from build123d import *

# Parameters (mm, degrees)
SKETCH_1_R          = 1.525
EXTRUDE_1_DEPTH     = 3.75
SKETCH_2_R          = 2.5
CUT_EXTRUDE_1_DEPTH = 10.5
CHAMFER_1_SIZE      = 3
SKETCH_3_R          = 2.5
CUT_EXTRUDE_2_DEPTH = 15.84082208
FILLET_1_R          = 0.5


with BuildPart() as part:
    # 草图1 → 凸台-拉伸1 (new, symmetric)
    with BuildSketch(Plane.XY):
        Polygon((-10, 8), (-10, -8), (6.931382282, -8), (10, -7), (10, 7), (6.931382282, 8), align=None)
        with Locations((0, 5)):
            Circle(SKETCH_1_R, mode=Mode.SUBTRACT)
        with Locations((0, -5)):
            Circle(SKETCH_1_R, mode=Mode.SUBTRACT)
    extrude(amount=EXTRUDE_1_DEPTH, both=True)

    # 草图2 → 切除-拉伸1 (cut)
    with BuildSketch(Plane.ZY.offset(10)):
        with Locations((4.25, 0)):
            Circle(SKETCH_2_R)
    extrude(amount=-CUT_EXTRUDE_1_DEPTH, mode=Mode.SUBTRACT)

    # 倒角1
    chamfer_1_edges = [part.edges().sort_by_distance(p)[0] for p in [
        (-10, -8, 0),
        (-10, 8, 0),
    ]]
    chamfer(chamfer_1_edges, length=CHAMFER_1_SIZE)

    # 草图3 → 切除-拉伸2 (cut, through all)
    with BuildSketch(Plane(origin=(0, 0, -3.75), x_dir=(-1, 0, 0), z_dir=(0, 0, -1))):
        with Locations((-10, 0)):
            Circle(SKETCH_3_R)
    extrude(amount=-CUT_EXTRUDE_2_DEPTH, mode=Mode.SUBTRACT)

    # 圆角1
    fillet_1_edges = [part.edges().sort_by_distance(p)[0] for p in [
        (6.931382282, 8, 0),
        (10, 7, 0),
        (10, -7, 0),
        (6.931382282, -8, 0),
        (-7, -8, 0),
        (-10, 5, 0),
        (-10, -5, 0),
        (-7, 8, 0),
        (10, -2.5, 0),
        (10, 2.5, 0),
    ]]
    fillet(fillet_1_edges, radius=FILLET_1_R)


solid = part.part
The model under review builds one solid part; all positions refer to its coordinate system, in mm. A direction names the side the tool comes from. Give positions to 0.01 mm unless a question says otherwise; leave off trailing zeros. Write each loop counter-clockwise with the first axis right and the second up, starting at its lowest first coordinate (ties: lowest second). Pieces come first, ordered by that corner, then holes.
1. Wall thickness on L1, parallel to Y at x = 0, z = 0 (3 decimals); L2, parallel to Y at x = -0.75, z = -2.75; L3, parallel to X at y = 0, z = -2.25: over which ranges is each line inside the solid? List them lowest first.
2. Tool access review of faces 1 (the flat face through (8.349, 7.538, 0.053)), 2 (the flat face through (0.5, 0, 3)): name each direction out of +Z, -Z, +X, -X, +Y, -Y from which nothing blocks a thin tool from reaching the whole face with its end or side.
3. For P1, Ø0.6, axis at y = -1, z = 3, coming from the -X side; P2, Ø1, axis at x = -3, y = 0, coming from the +Z side, all flat-tipped, find the tip position at first contact; note any pin that passes through.
4. Add section D-D, the plane y = 1.5. Write out the cut boundary in (x, z), plus the area to 3 significant figures.
5. Add section A-A, the plane x = 0. Write out the cut boundary in (y, z) (3 decimals).
6. Add section C-C, the plane z = 2.75. Write out the cut boundary in (x, y) (3 decimals).
7. Draft analysis for pull direction X (two halves, no side actions). For faces 3 (the cylindrical face through (-4.82, 0.05, 1.75)), 4 (the flat face through (10, -5, 0)), 5 (the flat face through (-8, 7, 0)), 6 (the cylindrical face through (0.8, -3.7, -0.1)), state which applies: +X half, -X half, draft (parallel to the pull), parting line (faces both ways), or undercut.
8. Add section B-B, the plane y = 4.25. Write out the cut boundary in (x, z).
Worked answers:
1. L1: y = -8 to -6.525, -3.475 to 3.475, 6.525 to 8
1. L2: y = -8 to -6.33, -3.67 to 3.67, 6.33 to 8
1. L3: x = -10 to 7.5
2. face 1: +Z, -Z, +X, +Y
2. face 2: +Z, -X
3. P1: stops at x = 0.5
3. P2: stops at z = 1.8
4. outline: (-10, -3.75) - (8, -3.75) - (8, 3.75) - (0.5, 3.75) - (0.5, 2.25) - (-10, 2.25) - close
4. area: 119 mm2
5. outline: (-8, -3.75) - (-6.525, -3.75) - (-6.525, 3.75) - (-8, 3.75) - close; (-3.475, -3.75) - (3.475, -3.75) - (3.475, 3.75) - (2.449, 3.75) arc R2.5 cw to (-2.449, 3.75) - (-3.475, 3.75) - close; (6.525, -3.75) - (8, -3.75) - (8, 3.75) - (6.525, 3.75) - close
6. outline: (-10, -4.793) arc R0.5 ccw to (-9.854, -5.146) - (-7.146, -7.854) arc R0.5 ccw to (-6.793, -8) - (6.852, -8) arc R0.5 ccw to (7.007, -7.975) - (9.655, -7.112) arc R0.5 ccw to (10, -6.637) - (10, -2.958) arc R0.5 ccw to (9.583, -2.465) arc R2.5 cw to (9.583, 2.465) arc R0.5 ccw to (10, 2.958) - (10, 6.637) arc R0.5 ccw to (9.655, 7.112) - (7.007, 7.975) arc R0.5 ccw to (6.852, 8) - (-6.793, 8) arc R0.5 ccw to (-7.146, 7.854) - (-9.854, 5.146) arc R0.5 ccw to (-10, 4.793) - (-10, 2) - (0.5, 2) - (0.5, -2) - (-10, -2) - close; hole circle Ø3.05 at (0, -5); hole circle Ø3.05 at (0, 5)
7. face 3: draft
7. face 4: +X half
7. face 5: -X half
7. face 6: undercut
8. outline: (-10, -3.75) - (-1.33, -3.75) - (-1.33, 3.75) - (-10, 3.75) - close; (1.33, -3.75) - (10, -3.75) - (10, 3.75) - (1.33, 3.75) - close
